```python
from build123d import *

# Parameters (mm, degrees)
F1_DEPTH  = 2.4
F2_W      = 40
F2_H      = 29
F3_DEPTH  = 2
F4_R      = 9.5
F4_R_2    = 3.5
F5_DEPTH  = 1.4
F6_DEPTH  = 4.4010001
F7_W      = 29
F7_H      = 29
F7_W_2    = 25
F7_H_2    = 25
F8_DEPTH  = 2.9
F9_W      = 29
F9_H      = 29
F9_W_2    = 22.8
F9_H_2    = 22.8
F10_DEPTH = 5
F11_F1_R  = 1
F11_F2_R  = 1
F12_SIZE  = 1.5
F13_R     = 0.5


with BuildPart() as f1:
    # F0 (on Top) → F1 (new body)
    with BuildSketch(Plane.XY):
        with BuildLine():
            Line((0, 11.8), (-4.8, 11.8))
            add(Edge.make_bspline(
                [(-4.8, 11.8), (-5.7190243266, 11.8), (-6.1421032596, 10.873414806), (-6.3, 10)],
                knots=[0, 0, 0, 0, 2.3430749028, 2.3430749028, 2.3430749028, 2.3430749028], degree=3))
            add(Edge.make_bspline(
                [(-6.3, 10), (-6.75, 6.8473730727), (-6.8, 3.4224423006), (-6.8, 0)],
                knots=[0, 0, 0, 0, 10.0124921973, 10.0124921973, 10.0124921973, 10.0124921973], degree=3))
            add(Edge.make_bspline(
                [(-6.3, -10), (-6.75, -6.8473730727), (-6.8, -3.4224423006), (-6.8, 0)],
                knots=[0, 0, 0, 0, 10.0124921973, 10.0124921973, 10.0124921973, 10.0124921973], degree=3))
            add(Edge.make_bspline(
                [(-4.8, -11.8), (-5.7190243266, -11.8), (-6.1421032596, -10.873414806), (-6.3, -10)],
                knots=[0, 0, 0, 0, 2.3430749028, 2.3430749028, 2.3430749028, 2.3430749028], degree=3))
            Line((-4.8, -11.8), (0, -11.8))
            Line((0, -11.8), (4.8, -11.8))
            add(Edge.make_bspline(
                [(4.8, -11.8), (5.7190243266, -11.8), (6.1421032596, -10.873414806), (6.3, -10)],
                knots=[0, 0, 0, 0, 2.3430749028, 2.3430749028, 2.3430749028, 2.3430749028], degree=3))
            add(Edge.make_bspline(
                [(6.3, -10), (6.75, -6.8473730727), (6.8, -3.4224423006), (6.8, 0)],
                knots=[0, 0, 0, 0, 10.0124921973, 10.0124921973, 10.0124921973, 10.0124921973], degree=3))
            add(Edge.make_bspline(
                [(6.3, 10), (6.75, 6.8473730727), (6.8, 3.4224423006), (6.8, 0)],
                knots=[0, 0, 0, 0, 10.0124921973, 10.0124921973, 10.0124921973, 10.0124921973], degree=3))
            add(Edge.make_bspline(
                [(4.8, 11.8), (5.7190243266, 11.8), (6.1421032596, 10.873414806), (6.3, 10)],
                knots=[0, 0, 0, 0, 2.3430749028, 2.3430749028, 2.3430749028, 2.3430749028], degree=3))
            Line((4.8, 11.8), (0, 11.8))
        make_face()
    extrude(amount=F1_DEPTH)

    # F2 (on face) → F3 (join)
    with BuildSketch(Plane.XY.offset(2.4)):
        Rectangle(F2_W, F2_H)
    extrude(amount=F3_DEPTH)

    # F4 (on face) → F5 (cut)
    with BuildSketch(Plane.XY.offset(4.4)):
        Circle(F4_R)
        Circle(F4_R_2, mode=Mode.SUBTRACT)
    extrude(amount=-F5_DEPTH, mode=Mode.SUBTRACT)

    # F6 (cut, through all): a face of the model
    f6_faces = [f1.faces().sort_by_distance(p)[0] for p in [
        (0, 0, 4.4),
    ]]
    extrude(f6_faces, amount=-F6_DEPTH, mode=Mode.SUBTRACT)

    # F7 (on face) → F8 (join)
    with BuildSketch(Plane.XY.offset(4.4)):
        Rectangle(F7_W, F7_H)
        Rectangle(F7_W_2, F7_H_2, mode=Mode.SUBTRACT)
    extrude(amount=F8_DEPTH)

    # F9 (on face) → F10 (join)
    with BuildSketch(Plane.XY.offset(7.3)):
        Rectangle(F9_W, F9_H)
        Rectangle(F9_W_2, F9_H_2, mode=Mode.SUBTRACT)
    extrude(amount=F10_DEPTH)

    # F11: fillet of radius 1 on 24 edges, made by hand

    # F11_f1
    f11_f1_edges = [f1.edges().sort_by_distance(p)[0] for p in [
        (12.5, -12.5, 5.85),
        (11.4, 11.4, 9.8),
        (12.5, 12.5, 5.85),
        (-12.5, -12.5, 5.85),
        (-11.4, -11.4, 9.8),
        (-12.5, 12.5, 5.85),
        (14.5, 0, 4.4),
        (-14.5, 0, 4.4),
        (11.4, -11.4, 9.8),
        (-11.4, 11.4, 9.8),
    ]]
    fillet(f11_f1_edges, radius=F11_F1_R)

    # F11_f2
    f11_f2_edges = [f1.edges().sort_by_distance(p)[0] for p in [
        (-20, -14.5, 3.4),
        (20, -14.5, 3.4),
        (14.5, -14.5, 8.85),
        (-14.5, -14.5, 8.85),
        (-14.5, 14.5, 8.85),
        (-20, 14.5, 3.4),
        (20, 14.5, 3.4),
        (14.5, 14.5, 8.85),
        (-20, 0, 4.4),
        (20, 0, 4.4),
        (14.5, 0, 12.3),
        (0, -14.5, 12.3),
        (-14.5, 0, 12.3),
        (0, 14.5, 12.3),
        (14.7928932188, 14.5, 4.6928932188),
        (-14.7928932188, 14.5, 4.6928932188),
        (-14.7928932188, -14.5, 4.6928932188),
        (14.7928932188, -14.5, 4.6928932188),
    ]]
    fillet(f11_f2_edges, radius=F11_F2_R)

    # F12
    f12_edges = [f1.edges().sort_by_distance(p)[0] for p in [
        (0, 11.4, 12.3),
    ]]
    chamfer(f12_edges, length=F12_SIZE)

    # F13
    f13_edges = [f1.edges().sort_by_distance(p)[0] for p in [
        (-6.722447, -5.009541, 0),
        (0, -11.8, 0),
        (0, 11.8, 0),
        (6.722447, 5.009541, 0),
    ]]
    fillet(f13_edges, radius=F13_R)


solid = f1.part
```
Verification items for the finished model (mm, model axes). A direction names the side the tool comes from. Round coordinates to 2 decimals unless told otherwise and drop trailing zeros. Loops run counter-clockwise (first coordinate to the right, second up) from the corner with the lowest first, then second, coordinate; pieces in that order, holes last. Notation, with made-up numbers: (36.5, 24) -> (42.5, 24) arc R11 cw to (42.5, 45) -> close; hole circle Ø1 at (18.5, 3). An arc over 180 degrees is marked (long way). Answer as a JSON object with one key per item and string values.
Q1. Section check B-B (z = 9.5). Record the boundary of the cut face in (x, y).
Data:
{"outline": "(-14.5, -13.5) arc R1 ccw to (-13.5, -14.5) -> (13.5, -14.5) arc R1 ccw to (14.5, -13.5) -> (14.5, 13.5) arc R1 ccw to (13.5, 14.5) -> (-13.5, 14.5) arc R1 ccw to (-14.5, 13.5) -> close; hole (-11.4, -10.4) arc R1 ccw to (-10.4, -11.4) -> (10.4, -11.4) arc R1 ccw to (11.4, -10.4) -> (11.4, 10.4) arc R1 ccw to (10.4, 11.4) -> (-10.4, 11.4) arc R1 ccw to (-11.4, 10.4) -> close"}
Q2. Section check D-D (x = -9). Record the boundary of the cut face in (y, z).
Data:
{"outline": "(-14.5, 2.4) -> (14.5, 2.4) -> (14.5, 11.3) arc R1 ccw to (13.5, 12.3) -> (12.9, 12.3) -> (11.4, 10.8) -> (11.4, 7.3) -> (12.5, 7.3) -> (12.5, 4.4) -> (3.04, 4.4) -> (3.04, 3) -> (-3.04, 3) -> (-3.04, 4.4) -> (-12.5, 4.4) -> (-12.5, 7.3) -> (-11.4, 7.3) -> (-11.4, 10.8) -> (-12.9, 12.3) -> (-13.5, 12.3) arc R1 ccw to (-14.5, 11.3) -> close"}
Q3. Access from +Z, -Z, +X, -X, +Y, -Y to the whole of each face (thin tool, end or side, straight path). Record for faces 4 (the flat face through (-14.5, 0, 8)), 5 (the flat face through (0, 11.4, 9)), 6 (the flat face through (0, 11.8, 1)).
Data:
{"face 4": "+Z, -X, +Y, -Y", "face 5": "+Z", "face 6": "-Z, +X, -X, +Y"}
Q4. Section check C-C (x = 17). Record the boundary of the cut face in (y, z), then the cut area to 3 significant figures.
Data:
{"outline": "(-14.5, 2.4) -> (14.5, 2.4) -> (14.5, 3.4) arc R1 ccw to (13.5, 4.4) -> (-13.5, 4.4) arc R1 ccw to (-14.5, 3.4) -> close", "area": "57.6 mm2"}
Q5. Scan lines: line 1 (Y direction, x = 0, z = 2.35); line 2 (Y direction, x = 0, z = 3.45); line 3 (X direction, y = -10.5, z = 9). Record each from-to range of solid material in increasing order. Write a range as from..to.
Data:
{"line 1": "y = -11.8..-3.5, 3.5..11.8", "line 2": "y = -14.5..-9.5, 9.5..14.5", "line 3": "x = -14.5..-11.39, 11.39..14.5"}
Q6. Go/stop test with flat-tipped pins: P1, Ø3, axis at y = -2.5, z = 8.5, coming from the +X side; P2, Ø6, axis at x = -14.5, z = 5.5, coming from the -Y side; P3, Ø1.5, axis at x = 0, z = 1, coming from the +Y side; P4, Ø1.1, axis at y = -0.5, z = 9, coming from the -X side. Record where each tip stops, or that it passes through.
Data:
{"P1": "stops at x = 14.5", "P2": "stops at y = -14.5", "P3": "stops at y = 11.8", "P4": "stops at x = -14.5"}
Q7. Draft check along X on faces 1 (the cylindrical face through (0.189, 14.215, 11.999)), 2 (the cylindrical face through (-19.699, 14.215, 2.907)), 3 (the flat face through (11.4, 0, 9)). Enter one of: pulls with the +X half, pulls with the -X half, needs draft (parallel to the pull), parting line crosses it, or undercut.
Data:
{"face 1": "needs draft", "face 2": "pulls with the -X half", "face 3": "undercut"}
